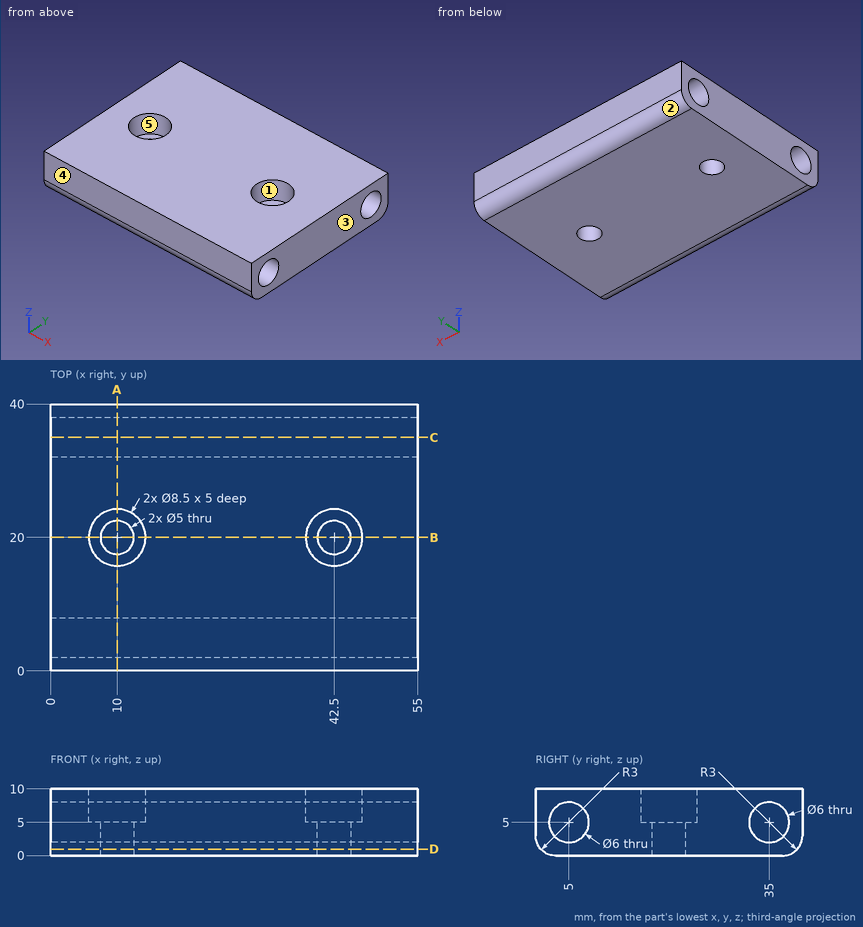
Here's the drawing with two shaded views (mm, measured from the low corner). I have some questions. A direction names the side the tool comes from. Coordinates: 2 decimals unless noted, no trailing zeros. Order: outer loops, then holes, each group sorted by start corner. A loop starts at its lowest first (then second) coordinate and runs counter-clockwise, first axis right, second up. Notation, with made-up numbers: (75, -28.75) - (133, -28.75) arc R21 cw to (133, -18.75) - close; hole circle Ø4 at (75.5, 58.25). An arc over 180 degrees is marked (long way). Answer in a Markdown table with one row per item. Add a question column.
(1) If we mould it in two halves opening along Y, with no side actions, what happens to the marked faces 1, 2 and 3? For each: released by +Y, released by -Y, zero draft, split by the parting line, or undercut.
(2) I need wall thicknesses on L1, parallel to X at y = 20, z = 7.7; L2, parallel to Y at x = 42.5, z = 3.25; L3, parallel to Y at x = 44.5, z = 3. Which ranges of each line are inside material? Lowest first, please.
(3) On a 3-axis mill with a long thin cutter (end or side, diameter ignored), from which of +Z, -Z, +X, -X, +Y, -Y can I reach the whole of each face in a straight line? I mean the marked faces 4 and 5. Say none if no direction works.
(4) If we section it at B-B, the plane y = 20: Please give me the cut outline in (x, z), then the cut area to 3 significant figures.
(5) If we section it at A-A, the plane x = 10: Please give me the cut outline in (y, z), then the cut area to 3 significant figures.
(6) If we section it at C-C, the plane y = 35: Please give me the cut outline in (x, z).
(7) If we section it at D-D, the plane z = 1: Please give me the cut outline in (x, y).
(8) Will this pin go through, and if not, where does the flat tip stop? pin 1 (4 mm diameter, centred on x = 11.5, y = 18.5, fed in from +Z).
Results are:
| question | item | result |
|---|---|---|
| 1 | face 1 | undercut |
| 1 | face 2 | released by +Y |
| 1 | face 3 | zero draft |
| 2 | L1 | x = 0 to 5.75, 14.25 to 38.25, 46.75 to 55 |
| 2 | L2 | y = 0 to 2.56, 7.44 to 17.5, 22.5 to 32.56, 37.44 to 40 |
| 2 | L3 | y = 0 to 2.76, 7.24 to 18.5, 21.5 to 32.76, 37.24 to 40 |
| 3 | face 4 | +Z, -Z, +X, -X, -Y |
| 3 | face 5 | +Z |
| 4 | outline | (0, 0) - (7.5, 0) - (7.5, 5) - (5.75, 5) - (5.75, 10) - (0, 10) - close; (12.5, 0) - (40, 0) - (40, 5) - (38.25, 5) - (38.25, 10) - (14.25, 10) - (14.25, 5) - (12.5, 5) - close; (45, 0) - (55, 0) - (55, 10) - (46.75, 10) - (46.75, 5) - (45, 5) - close |
| 4 | area | 415 mm2 |
| 5 | outline | (0, 3) arc R3 ccw to (3, 0) - (17.5, 0) - (17.5, 5) - (15.75, 5) - (15.75, 10) - (0, 10) - close; (22.5, 0) - (37, 0) arc R3 ccw to (40, 3) - (40, 10) - (24.25, 10) - (24.25, 5) - (22.5, 5) - close; hole circle Ø6 at (5, 5); hole circle Ø6 at (35, 5) |
| 5 | area | 272 mm2 |
| 6 | outline | (0, 0) - (55, 0) - (55, 2) - (0, 2) - close; (0, 8) - (55, 8) - (55, 10) - (0, 10) - close |
| 7 | outline | (0, 0.76) - (55, 0.76) - (55, 39.24) - (0, 39.24) - close; hole circle Ø5 at (10, 20); hole circle Ø5 at (42.5, 20) |
| 8 | pin 1 | stops at z = 5 |
